Part model, mm, in its own coordinate system. A direction names the side the tool comes from. Coordinates: 2 decimals unless noted, no trailing zeros. Loops run counter-clockwise (first coordinate to the right, second up) from the corner with the lowest first, then second, coordinate; pieces in that order, holes last. Notation, with made-up numbers: (-10, 18) - (11, 18) arc R18 ccw to (11, 24) - close; hole circle Ø2 at (-24.75, 10.25). An arc over 180 degrees is marked (long way). Use a Markdown table: item, result. Add a question column.
1. Band-saw the part on C-C, the plane x = 642. Give the cut face in (y, z), plus the area to 3 significant figures.
2. Wall check: probe 1 along Y at (x, z) = (641.5, -1); probe 2 along Z at (x, y) = (506.5, 138). Give the ranges that are in metal, low to high. Write a range as [from, to].
3. Band-saw the part on B-B, the plane y = 195. Give the cut face in (x, z), plus the area to 3 significant figures.
4. Drop a flat-ended pin along its axis: pin 1 (0.8 mm diameter, centred on x = 519, z = 168, fed in from +Y). Give the stop position or say it passes through.
5. Band-saw the part on A-A, the plane z = 139. Give the cut face in (x, y), plus the area to 3 significant figures.
6. Pull direction Z, two halves, no side cores. Call faces 1 (the flat face through (394, 83, 168.5)), 2 (the flat face through (394, -125, -2)), 3 (the flat face through (394, 83, -167.5)), 4 (the flat face through (394, 77, -168.5)): pulls with the +Z half, pulls with the -Z half, needs draft (parallel to the pull), parting line crosses it, or undercut.
7. 3-axis set-ups, long thin cutter, end or side, ignore diameter. For faces 5 (the flat face through (394, 285, 2)), 6 (the flat face through (394, -126, 2)), 7 (the flat face through (394, 77, 167.5)): which of +Z, -Z, +X, -X, +Y, -Y reach the whole face in a straight line?
from build123d import *

# Parameters (mm, degrees)
SKETCH1_W              = 800
SKETCH1_H              = 410
BOSS_EXTRUDE1_DEPTH    = 167.5
CONVERT_SOLID1_DEPTH   = 800
CONVERT_SOLID1_2_DEPTH = 800


# Read off the part's stored shape, not the designer's step: Convert-Solid1
with BuildPart() as part:
    # Sketch1 → Boss-Extrude1 (new, symmetric)
    with BuildSketch(Plane.XY):
        with Locations((400, 80)):
            Rectangle(SKETCH1_W, SKETCH1_H)
    extrude(amount=BOSS_EXTRUDE1_DEPTH, both=True)

    # Convert-Solid1 outline → Convert-Solid1 (cut)
    with BuildSketch(Plane.YZ):
        with BuildLine():
            Line((285, 167.5), (-124, 167.5))
            ThreePointArc((-124, 167.5), (-124.707106781, 167.207106781), (-125, 166.5))
            Line((-125, 166.5), (-125, -166.5))
            ThreePointArc((-125, -166.5), (-124.707106781, -167.207106781), (-124, -167.5))
            Line((-124, -167.5), (284, -167.5))
            ThreePointArc((284, -167.5), (284.707106781, -167.207106781), (285, -166.5))
            Line((285, -166.5), (285, 167.5))
        make_face()
    extrude(amount=CONVERT_SOLID1_DEPTH, mode=Mode.SUBTRACT)

    # Convert-Solid1 2 outline → Convert-Solid1 2 (add)
    with BuildSketch(Plane.YZ):
        with BuildLine():
            Line((-125, 167.5), (283.585786438, 167.5))
            Line((283.585786438, 167.5), (283.585786438, 168.5))
            Line((283.585786438, 168.5), (-124, 168.5))
            ThreePointArc((-124, 168.5), (-125.414213562, 167.914213562), (-126, 166.5))
            Line((-126, 166.5), (-126, -166.5))
            ThreePointArc((-126, -166.5), (-125.414213562, -167.914213562), (-124, -168.5))
            Line((-124, -168.5), (284, -168.5))
            ThreePointArc((284, -168.5), (285.414213562, -167.914213562), (286, -166.5))
            Line((286, -166.5), (286, 166.085786438))
            Line((286, 166.085786438), (285, 166.085786438))
            Line((285, 166.085786438), (285, -167.5))
            Line((285, -167.5), (-125, -167.5))
            Line((-125, -167.5), (-125, 167.5))
        make_face()
    extrude(amount=CONVERT_SOLID1_2_DEPTH)


solid = part.part
Geometry check:
| question | item | result |
|---|---|---|
| 1 | outline | (-126, -166.5) arc R2 ccw to (-124, -168.5) - (284, -168.5) arc R2 ccw to (286, -166.5) - (286, 166.09) - (285, 166.09) - (285, -166.5) arc R1 cw to (284, -167.5) - (-124, -167.5) arc R1 cw to (-125, -166.5) - (-125, 166.5) arc R1 cw to (-124, 167.5) - (283.59, 167.5) - (283.59, 168.5) - (-124, 168.5) arc R2 ccw to (-126, 166.5) - close |
| 1 | area | 1,490 mm^2 |
| 2 | probe 1 | y = [-126, -125], [285, 286] |
| 2 | probe 2 | z = [-168.5, -167.5], [167.5, 168.5] |
| 3 | outline | (0, -168.5) - (800, -168.5) - (800, -167.5) - (0, -167.5) - close; (0, 167.5) - (800, 167.5) - (800, 168.5) - (0, 168.5) - close |
| 3 | area | 1,600 mm^2 |
| 4 | pin 1 | stops at y = 283.59 |
| 5 | outline | (0, -126) - (800, -126) - (800, -125) - (0, -125) - close; (0, 285) - (800, 285) - (800, 286) - (0, 286) - close |
| 5 | area | 1,600 mm^2 |
| 6 | face 1 | pulls with the +Z half |
| 6 | face 2 | undercut |
| 6 | face 3 | undercut |
| 6 | face 4 | pulls with the -Z half |
| 7 | face 5 | +Z, +X, -X |
| 7 | face 6 | +Z, -Z, +X, -X, -Y |
| 7 | face 7 | +X, -X, +Y |
